```python
from build123d import *

# Parameters (mm, degrees)
SKETCH2_W          = 16
SKETCH2_H          = 16
CUT_EXTRUDE1_DEPTH = 40


with BuildPart() as part:
    # Sketch1 → Revolve1 (revolve)
    with BuildSketch(Plane.XY):
        Polygon((0, 0), (0, 4), (0.346410162, 4.6), (39.653589838, 4.6), (40, 4), (40, 0), align=None)
    revolve(axis=Axis((40, 0, 0), (-1, 0, 0)))

    # Sketch2 → Cut-Extrude1 (cut)
    with BuildSketch(Plane(origin=(0, 0, 0), x_dir=(0, 0, -1), z_dir=(1, 0, 0))):
        Rectangle(SKETCH2_W, SKETCH2_H)
        Polygon((-4, 2.309401077), (-4, -2.309401077), (0, -4.618802154), (4, -2.309401077), (4, 2.309401077), (0, 4.618802154), align=None, mode=Mode.SUBTRACT)
    extrude(amount=CUT_EXTRUDE1_DEPTH, mode=Mode.SUBTRACT)

    # Sketch3 → Cut-Revolve1 (revolve, cut)
    with BuildSketch(Plane.XY):
        Polygon((0, 0), (0, 2.5), (0.433, 2.067), (11.306616994, 2.067), (12.5, 0), align=None)
    revolve(axis=Axis((12.5, 0, 0), (-1, 0, 0)), mode=Mode.SUBTRACT)

    # Sketch4 → Cut-Revolve2 (revolve, cut)
    with BuildSketch(Plane.XY):
        Polygon((27.5, 0), (28.693383006, 2.067), (39.567, 2.067), (40, 2.5), (40, 0), align=None)
    revolve(axis=Axis((40, 0, 0), (-1, 0, 0)), mode=Mode.SUBTRACT)


solid = part.part
```
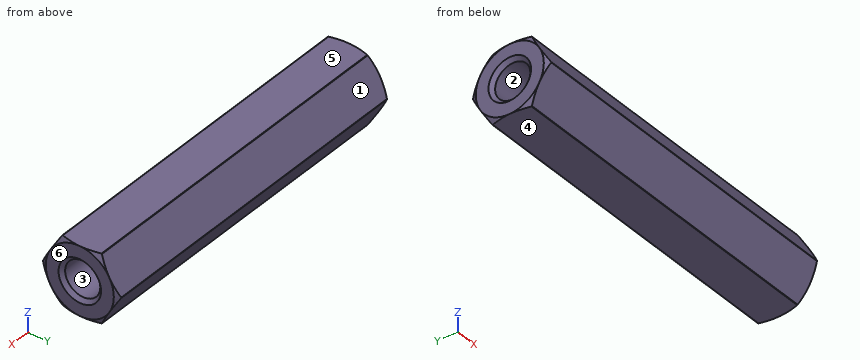
Design review of the part built by this model. Coordinates are the model's own, in mm. Face numbers are marked on the shaded views. A direction names the side the tool comes from. Coordinates: 2 decimals unless noted, no trailing zeros. Loops run counter-clockwise (first coordinate to the right, second up) from the corner with the lowest first, then second, coordinate; pieces in that order, holes last.
Q1. For pin 1 (1 mm diameter, centred on x = 19, y = 3.5, fed in from -Z); pin 2 (3.5 mm diameter, centred on y = 0, z = 0, fed in from +X); pin 3 (1.5 mm diameter, centred on x = 8, z = 3, fed in from -Y), all flat-tipped, find the tip position at first contact; note any pin that passes through.
Reported:
pin 1: stops at z = -2.8
pin 2: stops at x = 28.51
pin 3: stops at y = -3.32
Q2. The part is to be moulded in two halves that separate along Z. For the marked faces 3, 4, 5 and 6, say which applies: +Z half, -Z half, draft (parallel to the pull), parting line (faces both ways), or undercut.
Reported:
face 3: undercut
face 4: -Z half
face 5: +Z half
face 6: draft
Q3. To check wall thickness, follow line 1 (Y direction, x = 34.5, z = 0); line 2 (Z direction, x = 35.5, y = 0); line 3 (Z direction, x = 32.5, y = 0.5). State the ranges of each line that lie inside material, in increasing order.
Reported:
line 1: y = -4.6 to -2.07, 2.07 to 4.6
line 2: z = -4 to -2.07, 2.07 to 4
line 3: z = -4 to -2.01, 2.01 to 4
Q4. Tool access review of the marked faces 1 and 2: name each direction out of +Z, -Z, +X, -X, +Y, -Y from which nothing blocks a thin tool from reaching the whole face with its end or side.
Reported:
face 1: +Z, +X, -X, +Y
face 2: -X
Q5. We need section B-B on x = 18.5. State the section outline as (y, z) points, and give its area (3 significant figures).
Reported:
outline: (-4.6, -0.03) - (-2.33, -3.97) arc R4.6 ccw to (-2.27, -4) - (2.27, -4) arc R4.6 ccw to (2.33, -3.97) - (4.6, -0.03) arc R4.6 ccw to (4.6, 0.03) - (2.33, 3.97) arc R4.6 ccw to (2.27, 4) - (-2.27, 4) arc R4.6 ccw to (-2.33, 3.97) - (-4.6, 0.03) arc R4.6 ccw to start
area: 55.4 mm2
Q6. We need section A-A on x = 32. State the section outline as (y, z) points, and give its area (3 significant figures).
Reported:
outline: (-4.6, -0.03) - (-2.33, -3.97) arc R4.6 ccw to (-2.27, -4) - (2.27, -4) arc R4.6 ccw to (2.33, -3.97) - (4.6, -0.03) arc R4.6 ccw to (4.6, 0.03) - (2.33, 3.97) arc R4.6 ccw to (2.27, 4) - (-2.27, 4) arc R4.6 ccw to (-2.33, 3.97) - (-4.6, 0.03) arc R4.6 ccw to start; hole circle Ø4.13 at (0, 0)
area: 42.0 mm2
